The model under review builds one solid part; all positions refer to its coordinate system, in mm. A direction names the side the tool comes from. Round coordinates to 2 decimals unless told otherwise and drop trailing zeros. Order: outer loops, then holes, each group sorted by start corner. A loop starts at its lowest first (then second) coordinate and runs counter-clockwise, first axis right, second up. Notation, with made-up numbers: M -19.5,22 L -3.5,22 A23 cw -3.5,53 Z; hole C -34,75.25 d9. An arc over 180 degrees is marked long. Answer as a JSON object with one key per item and string values. Group by question number.
1. Add section A-A on z = -25.5. State the section outline as (x, y) points (3 decimals), and give its area (3 significant figures).
2. Add section B-B on x = 14. State the section outline as (y, z) points (3 decimals), and give its area (3 significant figures).
3. Machinability: for faces 1 (the face through (50.8, 2, 7)), 2 (the face through (-49, 2, 22.225)), 3 (the face through (47.498, 2, -51)), 4 (the face through (49, 2, 28.829)), which of the approach directions +Z, -Z, +X, -X, +Y, -Y give a long, thin tool a straight path to every point of the face, cutting with its end or side? Answer none if there is none.
4. To check wall thickness, follow probe 1 along X at (y, z) = (1.6, -1.5); probe 2 along Z at (x, y) = (-10, 2.7) (3 decimals). State the ranges of each line that lie inside material, in increasing order. Write a range as [from, to].
5. Mouldability with a two-part tool opening along X and no side actions: class faces 5 (the face through (-13, 2, 47.625)), 6 (the face through (-25, 2, 47.625)), 7 (the face through (-47.498, 2, 25)), 8 (the face through (49, 2, -3.175)) as released by +X, released by -X, zero draft, split by the parting line, or undercut.
6. Clearance check with flat-ended pins moving along their axes: P1, Ø1.6, axis at x = -49, y = 2.5, coming from the +Z side (3 decimals); P2, Ø3, axis at x = 38, z = -24, coming from the -Y side; P3, Ø1.6, axis at y = 1.5, z = 52, coming from the -X side; P4, Ø1.6, axis at y = 1, z = -25.5, coming from the -X side. State where each tip first meets the part, or that it passes through.
```python
from build123d import *

# Parameters (mm, degrees)
SKETCH1_W           = 101.6
SKETCH1_H           = 107.95
BOSS_EXTRUDE1_DEPTH = 3.175
SKETCH2_W           = 3.302
SKETCH2_H           = 6.604
CUT_EXTRUDE1_DEPTH  = 75.189091179


with BuildPart() as part:
    # Sketch1 → Boss-Extrude1 (new body)
    with BuildSketch(Plane(origin=(0, 0, 0), x_dir=(1, 0, 0), z_dir=(0, 1, 0))):
        Rectangle(SKETCH1_W, SKETCH1_H)
    extrude(amount=BOSS_EXTRUDE1_DEPTH)

    # Sketch2 → Cut-Extrude1 (cut, through all)
    with BuildSketch(Plane.XZ):
        Polygon((-34.798, 47.625), (-47.498, 47.625), (-50.8, 47.625), (-50.8, 54.229), (-50.8, 63.03162391), (50.8, 63.03162391), (50.8, 54.229), (50.8, 47.625), (47.498, 47.625), (34.671, 47.625), (34.671, 54.229), (28.702, 54.229), (28.702, 47.625), (21.971, 47.625), (21.971, 54.229), (16.002, 54.229), (16.002, 47.625), (9.271, 47.625), (9.271, 54.229), (3.302, 54.229), (3.302, 47.625), (-3.429, 47.625), (-3.429, 54.229), (-9.398, 54.229), (-9.398, 47.625), (-16.129, 47.625), (-16.129, 54.229), (-22.098, 54.229), (-22.098, 47.625), (-28.829, 47.625), (-28.829, 54.229), (-34.798, 54.229), align=None)
        with Locations((49.149, 38.227)):
            Rectangle(SKETCH2_W, SKETCH2_H)
        with Locations((49.149, 25.527)):
            Rectangle(SKETCH2_W, SKETCH2_H)
        with Locations((49.149, 12.827)):
            Rectangle(SKETCH2_W, SKETCH2_H)
        with Locations((49.149, 0.127)):
            Rectangle(SKETCH2_W, SKETCH2_H)
        with Locations((49.149, -12.573)):
            Rectangle(SKETCH2_W, SKETCH2_H)
        with Locations((49.149, -25.273)):
            Rectangle(SKETCH2_W, SKETCH2_H)
        with Locations((49.149, -37.973)):
            Rectangle(SKETCH2_W, SKETCH2_H)
        with Locations((-49.149, -37.973)):
            Rectangle(SKETCH2_W, SKETCH2_H)
        with Locations((-49.149, -25.273)):
            Rectangle(SKETCH2_W, SKETCH2_H)
        with Locations((-49.149, -12.573)):
            Rectangle(SKETCH2_W, SKETCH2_H)
        with Locations((-49.149, 0.127)):
            Rectangle(SKETCH2_W, SKETCH2_H)
        with Locations((-49.149, 12.827)):
            Rectangle(SKETCH2_W, SKETCH2_H)
        with Locations((-49.149, 25.527)):
            Rectangle(SKETCH2_W, SKETCH2_H)
        with Locations((-49.149, 38.227)):
            Rectangle(SKETCH2_W, SKETCH2_H)
        with Locations((49.149, -50.673)):
            Rectangle(SKETCH2_W, SKETCH2_H)
        with Locations((-49.149, -50.673)):
            Rectangle(SKETCH2_W, SKETCH2_H)
    extrude(amount=-CUT_EXTRUDE1_DEPTH, mode=Mode.SUBTRACT)


solid = part.part
```
Recorded:
{
 "1": {"outline": "M -47.498,0 L 47.498,0 L 47.498,3.175 L -47.498,3.175 Z", "area": "302 mm²"},
 "2": {"outline": "M 0,-53.975 L 3.175,-53.975 L 3.175,47.625 L 0,47.625 Z", "area": "323 mm²"},
 "3": {"face 1": "+Z, -Z, +X, +Y, -Y", "face 2": "-X, +Y, -Y", "face 3": "-Z, +X, +Y, -Y", "face 4": "+X, +Y, -Y"},
 "4": {"probe 1": "x = [-47.5, 47.5]", "probe 2": "z = [-53.975, 47.625]"},
 "5": {"face 5": "undercut", "face 6": "undercut", "face 7": "released by -X", "face 8": "zero draft"},
 "6": {"P1": "stops at z = 47.625", "P2": "stops at y = 0", "P3": "stops at x = -34.8", "P4": "stops at x = -47.5"}
}
